Part model, mm, in its own coordinate system. A direction names the side the tool comes from. Give positions to 0.01 mm unless a question says otherwise; leave off trailing zeros. Loops run counter-clockwise (first coordinate to the right, second up) from the corner with the lowest first, then second, coordinate; pieces in that order, holes last. Notation, with made-up numbers: (62, 77) -> (95, 77) arc R31 ccw to (95, 101) -> close; hole circle Ø6 at (57, 80.25). An arc over 180 degrees is marked (long way). Write item = value, one per line.
from build123d import *

# Parameters (mm, degrees)
F0_W      = 58.2
F0_H      = 58.2
F1_DEPTH  = 76
F2_R      = 2.5
F3_DEPTH  = 25
F4_W      = 154.9799069762
F4_H      = 154.0232300758
F5_DEPTH  = 71
F6_R      = 1
F7_R      = 3
F8_R      = 19.05
F9_DEPTH  = 1.6
F10_R     = 3.175
F11_DEPTH = 18.5
F13_DEPTH = 15
F14_R     = 3.175
F15_DEPTH = 15


with BuildPart() as f1:
    # F0 (on Front) → F1 (new body)
    with BuildSketch(Plane.XZ):
        Rectangle(F0_W, F0_H)
    extrude(amount=F1_DEPTH)

    # F2 (on face) → F3 (cut)
    with BuildSketch(Plane.XZ.offset(76)):
        with Locations((23.55, 23.55)):
            Circle(F2_R)
        with Locations((23.55, -23.55)):
            Circle(F2_R)
        with Locations((-23.55, -23.55)):
            Circle(F2_R)
        with Locations((-23.55, 23.55)):
            Circle(F2_R)
    extrude(amount=-F3_DEPTH, mode=Mode.SUBTRACT)

    # F4 (on face) → F5 (cut)
    with BuildSketch(Plane(origin=(0, 0, 0), x_dir=(-1, 0, 0), z_dir=(0, 1, 0))):
        with Locations((-0.8317120373, 1.2900978327)):
            Rectangle(F4_W, F4_H)
        with BuildLine():
            Line((27.330764838, 19.555526663), (46.886291501, 0))
            Line((46.886291501, 0), (27.330764838, -19.555526663))
            ThreePointArc((27.330764838, -19.555526663), (19.6609127035, -19.6609127035), (19.555526663, -27.330764838))
            Line((19.555526663, -27.330764838), (0, -46.886291501))
            Line((0, -46.886291501), (-19.555526663, -27.330764838))
            ThreePointArc((-19.555526663, -27.330764838), (-19.6609127035, -19.6609127035), (-27.330764838, -19.555526663))
            Line((-27.330764838, -19.555526663), (-46.886291501, 0))
            Line((-46.886291501, 0), (-27.330764838, 19.555526663))
            ThreePointArc((-27.330764838, 19.555526663), (-19.6609127035, 19.6609127035), (-19.555526663, 27.330764838))
            Line((-19.555526663, 27.330764838), (0, 46.886291501))
            Line((0, 46.886291501), (19.555526663, 27.330764838))
            ThreePointArc((19.555526663, 27.330764838), (19.6609127035, 19.6609127035), (27.330764838, 19.555526663))
        make_face(mode=Mode.SUBTRACT)
    extrude(amount=-F5_DEPTH, mode=Mode.SUBTRACT)

    # F6
    f6_edges = [f1.edges().sort_by_distance(p)[0] for p in [
        (-29.1, -35.5, 17.786292),
        (-17.786292, -35.5, 29.1),
        (-19.555527, -35.5, 27.330765),
        (-27.330765, -35.5, 19.555527),
        (-29.1, -35.5, -17.786292),
        (-27.330765, -35.5, -19.555527),
        (-17.786292, -35.5, -29.1),
        (-19.555527, -35.5, -27.330765),
        (17.786292, -35.5, -29.1),
        (19.555527, -35.5, -27.330765),
        (27.330765, -35.5, -19.555527),
        (29.1, -35.5, -17.786292),
        (27.330765, -35.5, 19.555527),
        (29.1, -35.5, 17.786292),
        (19.555527, -35.5, 27.330765),
        (17.786292, -35.5, 29.1),
    ]]
    fillet(f6_edges, radius=F6_R)

    # F7
    f7_edges = [f1.edges().sort_by_distance(p)[0] for p in [
        (-29.1, -73.5, -29.1),
        (-29.1, -73.5, 29.1),
        (29.1, -73.5, -29.1),
        (29.1, -73.5, 29.1),
    ]]
    fillet(f7_edges, radius=F7_R)

    # F8 (on face) → F9 (join)
    with BuildSketch(Plane.XZ.offset(76)):
        Circle(F8_R)
    extrude(amount=F9_DEPTH)

    # F10 (on face) → F11 (join)
    with BuildSketch(Plane.XZ.offset(77.6)):
        Circle(F10_R)
    extrude(amount=F11_DEPTH)

    # F12 (on face) → F13 (cut)
    with BuildSketch(Plane.XZ.offset(96.1)):
        with BuildLine():
            ThreePointArc((3.175, 0), (2.8662366441, 1.365764438), (2, 2.4658923334))
            Line((2, 2.4658923334), (2, -2.4658923334))
            ThreePointArc((2, -2.4658923334), (2.8662366441, -1.365764438), (3.175, 0))
        make_face()
    extrude(amount=-F13_DEPTH, mode=Mode.SUBTRACT)

    # F14 (on face) → F15 (join)
    with BuildSketch(Plane(origin=(0, 0, 0), x_dir=(-1, 0, 0), z_dir=(0, 1, 0))):
        Circle(F14_R)
    extrude(amount=F15_DEPTH)


solid = f1.part
1) Slice it at C-C, the plane z = 6.5. List the corners of the cut face in (x, y), and give its area (3 significant figures).
Resolved:
outline = (-29.1, -76) -> (-17.91, -76) -> (-17.91, -77.6) -> (17.91, -77.6) -> (17.91, -76) -> (29.1, -76) -> (29.1, 0) -> (-29.1, 0) -> close
area = 4,480 mm²
2) Slice it at B-B, the plane z = -23.55. List the corners of the cut face in (x, y), and give its area (3 significant figures).
Resolved:
outline = (-29.1, -76) -> (-26.05, -76) -> (-26.05, -71) -> (-29.1, -71) -> close; (-21.05, -76) -> (21.05, -76) -> (21.05, -71) -> (18.05, -71) -> (18.05, 0) -> (-18.05, 0) -> (-18.05, -71) -> (-21.05, -71) -> close; (26.05, -76) -> (29.1, -76) -> (29.1, -71) -> (26.05, -71) -> close
area = 2,800 mm²
3) Pull direction X, two halves, no side cores. Call faces 1 (the face through (-3.17, -86.72, 0.14)), 2 (the face through (4, -77.6, 0)), 3 (the face through (23.01, -73.54, -25.99)): pulls with the +X half, pulls with the -X half, needs draft (parallel to the pull), parting line crosses it, or undercut.
Resolved:
face_1 = parting line crosses it
face_2 = needs draft
face_3 = undercut
4) Slice it at A-A, the plane x = 23.55. List the corners of the cut face in (y, z).
Resolved:
outline = (-76, -29.1) -> (-71, -29.1) -> (-71, -26.05) -> (-76, -26.05) -> close; (-76, -21.05) -> (-71, -21.05) -> (-71, -18.05) -> (0, -18.05) -> (0, 18.05) -> (-71, 18.05) -> (-71, 21.05) -> (-76, 21.05) -> close; (-76, 26.05) -> (-71, 26.05) -> (-71, 29.1) -> (-76, 29.1) -> close
5) Slice it at D-D, the plane x = 0. List the corners of the cut face in (y, z) (3 decimals), and give its area (3 significant figures).
Resolved:
outline = (-96.1, -3.175) -> (-77.6, -3.175) -> (-77.6, -19.05) -> (-76, -19.05) -> (-76, -29.1) -> (0, -29.1) -> (0, -3.175) -> (15, -3.175) -> (15, 3.175) -> (0, 3.175) -> (0, 29.1) -> (-76, 29.1) -> (-76, 19.05) -> (-77.6, 19.05) -> (-77.6, 3.175) -> (-96.1, 3.175) -> close
area = 4,700 mm²
6) Drill centre lines: line 1 along Z through (x, y) = (-23.55, -74.15); line 2 along X through (y, z) = (-42, 19); line 3 along X through (y, z) = (-74, -23). Where is each one in solid material? Low to high. Write a range as [from, to].
Resolved:
line_1 = [-29.1, -26.05], [-21.05, 21.05], [26.05, 29.1]
line_2 = [-27.88, -26.64], [-20.46, 20.46], [26.64, 27.88]
line_3 = [-29.1, -25.99], [-21.11, 21.11], [25.99, 29.1]
7) Which spindle directions (+Z, -Z, +X, -X, +Y, -Y) get a long thin tool onto all of the face, cutting with end or side? Do faces 4 (the face through (2, -89, 0)), 5 (the face through (19.586, -35.003, -19.737)), 6 (the face through (-15.12, -76.79, -11.59)). Say none if no direction does.
Resolved:
face_4 = +Z, -Z, +X, -Y
face_5 = +Y
face_6 = -Y
8) Drop flat-ended pins along their axis: P1, Ø3, axis at x = 13.5, z = 7.5, coming from the +Y side; P2, Ø3, axis at x = -10.5, y = -80, coming from the -Z side; P3, Ø5, axis at x = 15, z = 17.5, coming from the -Y side; P4, Ø8, axis at x = -23.55, z = -23.55, coming from the +Y side. Give the stop position or say it passes through.
Resolved:
P1 = 0
P2 = through
P3 = -76
P4 = -71
